Verification items for the finished model (mm, model axes). A direction names the side the tool comes from. Coordinates: 2 decimals unless noted, no trailing zeros. Order: outer loops, then holes, each group sorted by start corner. A loop starts at its lowest first (then second) coordinate and runs counter-clockwise, first axis right, second up.
Q1. Draft check along Y on faces 5 (the cylindrical face through (9.17, 7.05, 25.63)), 6 (the flat face through (0, -6.35, 17)), 7 (the flat face through (1.5, 13, 24)). Enter one of: pulls with the +Y half, pulls with the -Y half, needs draft (parallel to the pull), parting line crosses it, or undercut.
Q2. Cross-section at C-C, the plane x = 10. Record the boundary of the cut face in (y, z).
Q3. Cross-section at A-A, the plane y = -4. Record the boundary of the cut face in (x, z), and give its area (3 significant figures).
Q4. Cross-section at D-D, the plane z = 12.5. Record the boundary of the cut face in (x, y), and give its area (3 significant figures).
Q5. Depth check by flat-ended pin: P1, Ø2.5, axis at x = 6.5, z = 18, coming from the +Y side; P2, Ø5, axis at x = 8.5, y = 5, coming from the -Z side; P3, Ø4.5, axis at y = 10.5, z = 27.5, coming from the -X side; P4, Ø5, axis at x = -10.5, z = 25.5, coming from the -Y side. Enter the tip coordinate at first touch or a pass-through.
Q6. Cross-section at B-B, the plane z = 25.5. Record the boundary of the cut face in (x, y), and give its area (3 significant figures).
Q7. Thickness scan on line 1 (Y direction, x = -5.25, z = 25.5); line 2 (X direction, y = 0, z = 27.25); line 3 (Z direction, x = 11, y = 5). Record the ranges inside material, lowest first.
Q8. Set-up check for faces 1 (the flat face through (9, 4, 19)), 2 (the cylindrical face through (-1.38, -6.2, 7.89)), 3 (the flat face through (-1.5, 9.5, 27)), 4 (the cylindrical face through (3.965, 11.178, 27.503)): record each of +Z, -Z, +X, -X, +Y, -Y from which the full face is reachable in a straight line by a thin tool's end or side.
from build123d import *

# Parameters (mm, degrees)
SKETCH1_R               = 15
SKETCH1_R_2             = 6.35
BOSS_EXTRUDE1_DEPTH     = 32
CUT_EXTRUDE1_DEPTH      = 16
CUT_EXTRUDE2_START      = -21.35
SKETCH3_W               = 30
SKETCH3_H               = 3
CUT_EXTRUDE2_DEPTH      = 21.274812
SKETCH4_R               = 1.65
CUT_EXTRUDE3_DEPTH      = 17.5
CUT_EXTRUDE3_DEPTH_BACK = 14.5
SKETCH5_R               = 2.1
CUT_EXTRUDE4_DEPTH      = 14.5000001
SKETCH6_R               = 3.5
CUT_EXTRUDE5_DEPTH      = 8.5


with BuildPart() as part:
    # Sketch1 → Boss-Extrude1 (new body)
    with BuildSketch(Plane.XY):
        Circle(SKETCH1_R)
        Circle(SKETCH1_R_2, mode=Mode.SUBTRACT)
    extrude(amount=BOSS_EXTRUDE1_DEPTH)

    # Sketch2 → Cut-Extrude1 (cut)
    with BuildSketch(Plane.XY.offset(32)):
        with BuildLine():
            Line((-1.5, 6.170291727), (-1.5, 14.924811557))
            ThreePointArc((-1.5, 14.924811557), (0, 16.424811557), (1.5, 14.924811557))
            Line((1.5, 14.924811557), (1.5, 6.170291727))
            ThreePointArc((1.5, 6.170291727), (0, 4.670291727), (-1.5, 6.170291727))
        make_face()
    extrude(amount=-CUT_EXTRUDE1_DEPTH, mode=Mode.SUBTRACT)

    # Sketch3 → Cut-Extrude2 (cut)
    with BuildSketch(Plane(origin=(0, 15, 0), x_dir=(1, 0, 0), z_dir=(0, 1, 0)).offset(CUT_EXTRUDE2_START)):
        with Locations((0, -17.5)):
            Rectangle(SKETCH3_W, SKETCH3_H)
    extrude(amount=CUT_EXTRUDE2_DEPTH, mode=Mode.SUBTRACT)

    # Sketch4 → Cut-Extrude3 (cut, two sides)
    with BuildSketch(Plane(origin=(-1.5, 0, 0), x_dir=(0, 0, -1), z_dir=(1, 0, 0))) as cut_extrude3_sk:
        with Locations((-25.5, 10.547551642)):
            Circle(SKETCH4_R)
    extrude(amount=CUT_EXTRUDE3_DEPTH, mode=Mode.SUBTRACT)
    extrude(cut_extrude3_sk.sketch, amount=-CUT_EXTRUDE3_DEPTH_BACK, mode=Mode.SUBTRACT)

    # Sketch5 → Cut-Extrude4 (cut, through all)
    with BuildSketch(Plane.ZY.offset(-1.5)):
        with Locations((25.5, 10.547551642)):
            Circle(SKETCH5_R)
    extrude(amount=-CUT_EXTRUDE4_DEPTH, mode=Mode.SUBTRACT)

    # Sketch6 → Cut-Extrude5 (cut)
    with BuildSketch(Plane(origin=(15, 0, 0), x_dir=(0, 0, -1), z_dir=(1, 0, 0))):
        with Locations((-25.5, 10.547551642)):
            Circle(SKETCH6_R)
    extrude(amount=-CUT_EXTRUDE5_DEPTH, mode=Mode.SUBTRACT)


solid = part.part
Check values:
1. face 5: undercut
1. face 6: pulls with the +Y half
1. face 7: needs draft
2. outline: (-11.18, 0) - (11.18, 0) - (11.18, 16) - (-6.35, 16) - (-6.35, 19) - (11.18, 19) - (11.18, 22.06) arc R3.5 cw (long way) to (11.18, 28.94) - (11.18, 32) - (-11.18, 32) - close
3. outline: (-14.46, 0) - (-4.93, 0) - (-4.93, 16) - (-14.46, 16) - close; (-14.46, 19) - (-4.93, 19) - (-4.93, 32) - (-14.46, 32) - close; (4.93, 0) - (14.46, 0) - (14.46, 16) - (4.93, 16) - close; (4.93, 19) - (14.46, 19) - (14.46, 32) - (4.93, 32) - close
3. area: 552 mm2
4. outline: circle Ø30 at (0, 0); hole circle Ø12.7 at (0, 0)
4. area: 580 mm2
5. P1: stops at y = 13.85
5. P2: stops at z = 0
5. P3: stops at x = -12.53
5. P4: stops at y = -12.69
6. outline: (-12.08, 8.9) arc R15 ccw (long way) to (13.24, 7.05) - (6.5, 7.05) - (6.5, 8.45) - (1.5, 8.45) - (1.5, 6.17) arc R6.35 cw (long way) to (-1.5, 6.17) - (-1.5, 8.9) - close; (-8.73, 12.2) - (-1.5, 12.2) - (-1.5, 14.92) arc R15 ccw to start; (1.5, 12.65) - (6.5, 12.65) - (6.5, 13.52) arc R15 ccw to (1.5, 14.92) - close
6. area: 477 mm2
7. line 1: y = -14.05 to -3.57, 3.57 to 8.9, 12.2 to 14.05
7. line 2: x = -15 to -6.35, 6.35 to 15
7. line 3: z = 0 to 16, 19 to 32
8. face 1: +X, -X, +Y
8. face 2: +Z, -Z
8. face 3: +Z, +Y
8. face 4: +X
